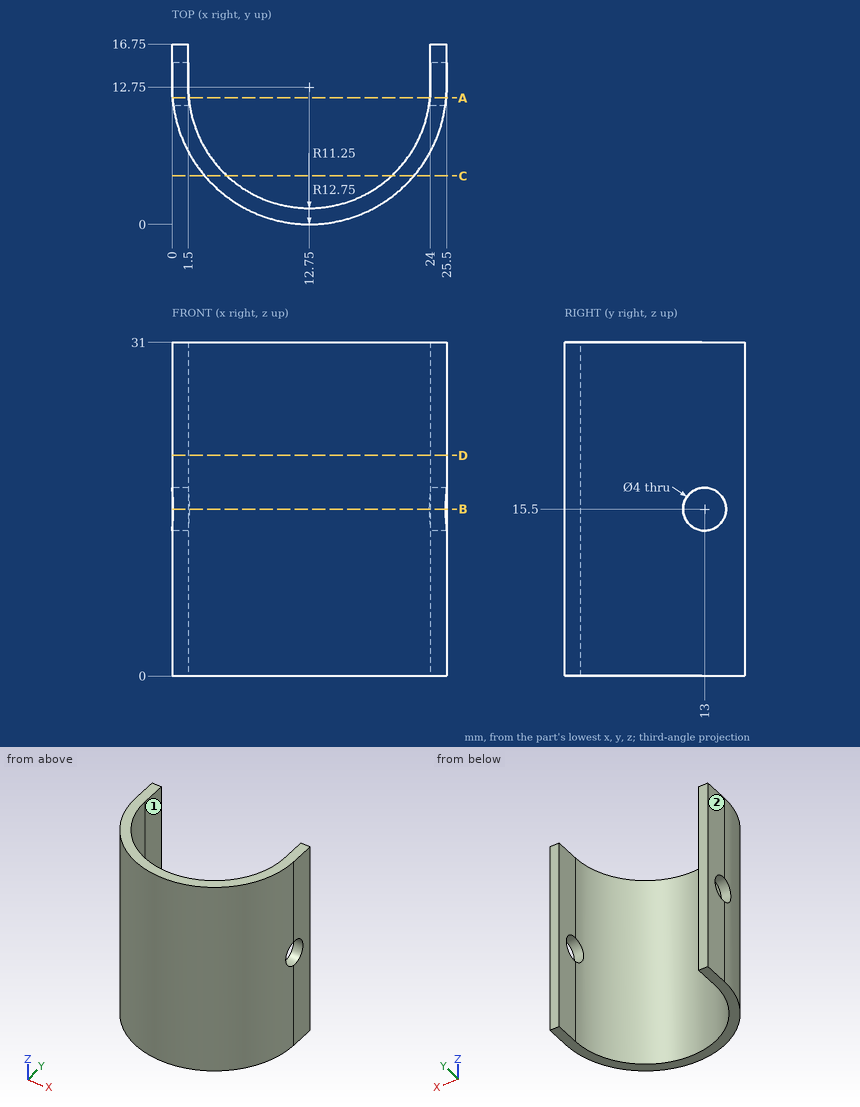
Geometry check sheet. Reference: drawing and pictorial views, mm from the part's lowest x, y, z. A direction names the side the tool comes from. Coordinates: 2 decimals unless noted, no trailing zeros. Write each loop counter-clockwise with the first axis right and the second up, starting at its lowest first coordinate (ties: lowest second). Pieces come first, ordered by that corner, then holes.
Item 1: Cross-section at C-C on y = 4.5. Record the boundary of the cut face in (x, z), then the cut area to 4 significant figures.
Numbers:
outline: (3.03, 0) - (5.1, 0) - (5.1, 31) - (3.03, 31) - close; (20.4, 0) - (22.47, 0) - (22.47, 31) - (20.4, 31) - close
area: 128.5 mm2
Item 2: Access from +Z, -Z, +X, -X, +Y, -Y to the whole of each face (thin tool, end or side, straight path). Record for the marked faces 1 and 2.
Numbers:
face 1: +Z, -Z, +Y
face 2: +Z, -Z, -X, +Y, -Y
Item 3: Depth check by flat-ended pin: pin 1 Ø5 at (y, z) = (5, 19.5) entering from -X; pin 2 Ø6 at (x, z) = (19, 6.5) entering from -Y; pin 3 Ø8 at (x, y) = (10.5, 4) entering from +Z; pin 4 Ø1 at (y, z) = (8.5, 20.5) entering from -X. Enter the tip coordinate at first touch or a pass-through.
Numbers:
pin 1: stops at x = 1.13
pin 2: stops at y = 0.42
pin 3: stops at z = 31
pin 4: stops at x = 0.56
Item 4: Cross-section at A-A on y = 11.75. Record the boundary of the cut face in (x, z), then the cut area to 3 significant figures.
Numbers:
outline: (0.04, 0) - (1.54, 0) - (1.54, 13.94) - (0.04, 13.94) - close; (0.04, 17.06) - (1.54, 17.06) - (1.54, 31) - (0.04, 31) - close; (23.96, 0) - (25.46, 0) - (25.46, 13.94) - (23.96, 13.94) - close; (23.96, 17.06) - (25.46, 17.06) - (25.46, 31) - (23.96, 31) - close
area: 83.9 mm2
Item 5: Cross-section at B-B on z = 15.5. Record the boundary of the cut face in (x, y).
Numbers:
outline: (0, 15) - (1.5, 15) - (1.5, 16.75) - (0, 16.75) - close; (0.12, 11) arc R12.75 ccw to (25.38, 11) - (23.86, 11) arc R11.25 cw to (1.64, 11) - close; (24, 15) - (25.5, 15) - (25.5, 16.75) - (24, 16.75) - close
Item 6: Cross-section at D-D on z = 20.5. Record the boundary of the cut face in (x, y).
Numbers:
outline: (0, 12.75) arc R12.75 ccw to (25.5, 12.75) - (25.5, 16.75) - (24, 16.75) - (24, 12.75) arc R11.25 cw to (1.5, 12.75) - (1.5, 16.75) - (0, 16.75) - close
Item 7: Scan lines: probe 1 along Z at (x, y) = (0.9, 13); probe 2 along X at (y, z) = (15.75, 19.5); probe 3 along X at (y, z) = (10.5, 20). Record each from-to range of solid material in increasing order.
Numbers:
probe 1: z = 0 to 13.5, 17.5 to 31
probe 2: x = 0 to 1.5, 24 to 25.5
probe 3: x = 0.2 to 1.73, 23.77 to 25.3
